from build123d import *

# Parameters (mm, degrees)
BOSS_EXTRUDE1_DEPTH = 15
DIAMETER_HOLE1_D    = 5.5
CHAMFER1_SIZE       = 5


with BuildPart() as part:
    # Sketch1 → Boss-Extrude1 (new body)
    with BuildSketch(Plane.XY):
        Polygon((-16, 36), (16, 36), (16, 10), (28, 10), (28, 0), (-28, 0), (-28, 10), (-16, 10), align=None)
    extrude(amount=-BOSS_EXTRUDE1_DEPTH)

    # Sketch2 → Cut-Revolve1 (revolve, cut)
    with BuildSketch(Plane(origin=(0, 0, 0), x_dir=(0, 0, -1), z_dir=(1, 0, 0)), mode=Mode.PRIVATE) as cut_revolve1_sk:
        Polygon((3.65, 32), (3.65, 32.6), (5, 32.6), (5, 32), (13, 32), (13, 30), (15, 30), (15, 20), (0, 20), (0, 32), align=None)
    revolve(cut_revolve1_sk.sketch.rotate(Axis((0, 20, -15), (0, 0, 1)), 90), axis=Axis((0, 20, -15), (0, 0, 1)), mode=Mode.SUBTRACT)

    # Diameter Hole1 (through all)
    with Locations(Plane(origin=(0, 10, 0), x_dir=(1, 0, 0), z_dir=(0, 1, 0))):
        with Locations((-22, 7.5), (22, 7.5)):
            Hole(DIAMETER_HOLE1_D / 2)

    # Chamfer1
    chamfer1_edges = [part.edges().sort_by_distance(p)[0] for p in [
        (-16, 36, -7.5),
        (16, 36, -7.5),
    ]]
    chamfer(chamfer1_edges, length=CHAMFER1_SIZE)


solid = part.part
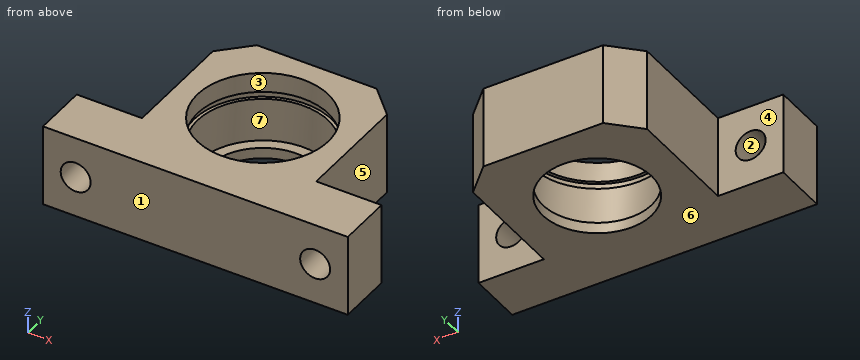
Can you work these out from the model? Positions are in its coordinate system, mm. Face numbers are marked on the shaded views. A direction names the side the tool comes from. Give positions to 0.01 mm unless a question says otherwise; leave off trailing zeros. Loops run counter-clockwise (first coordinate to the right, second up) from the corner with the lowest first, then second, coordinate; pieces in that order, holes last. Notation, with made-up numbers: (-14.75, 25.25) -> (-0.75, 25.25) arc R17 cw to (-0.75, 32.25) -> close; hole circle Ø3 at (28, 1). An arc over 180 degrees is marked (long way). Write item = value, one per line.
1) Suppose I cut it at D-D on y = 3.5. Write out the boundary of the cut face in (x, z).
Check result:
outline = (-28, -15) -> (28, -15) -> (28, 0) -> (-28, 0) -> close; hole circle Ø5.5 at (-22, -7.5); hole circle Ø5.5 at (22, -7.5)
2) Will these pins go through, and if not, where does the flat tip stop? pin 1 (6 mm diameter, centred on x = 24.5, z = -4.5, fed in from +Y); pin 2 (2 mm diameter, centred on y = 11.5, z = -5.5, fed in from -X); pin 3 (4 mm diameter, centred on y = 15.5, z = -5, fed in from +X).
Check result:
pin_1 = 10
pin_2 = -16
pin_3 = 16
3) Suppose I cut it at B-B on x = 22. Write out the boundary of the cut face in (y, z).
Check result:
outline = (0, -15) -> (10, -15) -> (10, -10.25) -> (0, -10.25) -> close; (0, -4.75) -> (10, -4.75) -> (10, 0) -> (0, 0) -> close
4) Suppose I cut it at A-A on z = -7.5. Write out the boundary of the cut face in (x, y).
Check result:
outline = (-28, 0) -> (-24.75, 0) -> (-24.75, 10) -> (-28, 10) -> close; (-19.25, 0) -> (19.25, 0) -> (19.25, 10) -> (16, 10) -> (16, 31) -> (11, 36) -> (-11, 36) -> (-16, 31) -> (-16, 10) -> (-19.25, 10) -> close; (24.75, 0) -> (28, 0) -> (28, 10) -> (24.75, 10) -> close; hole circle Ø24 at (0, 20)
5) For the marked faces 4, 5, 6 and 7, which set-ups out of +Z, -Z, +X, -X, +Y, -Y let a thin tool reach every point of the face, with its end or its side?
Check result:
face_4 = +Z, -Z, -X, +Y
face_5 = +Z, -Z, +X, +Y
face_6 = -Z, +X, -X, +Y, -Y
face_7 = +Z
6) Suppose I cut it at C-C on z = -2.25. Write out the boundary of the cut face in (x, y), then the cut area to 3 significant figures.
Check result:
outline = (-28, 0) -> (28, 0) -> (28, 10) -> (16, 10) -> (16, 31) -> (11, 36) -> (-11, 36) -> (-16, 31) -> (-16, 10) -> (-28, 10) -> close; hole circle Ø24 at (0, 20)
area = 915 mm2
7) I need wall thicknesses on L1, parallel to X at y = 20, z = -4.45; L2, parallel to Z at x = -22, y = 7; L3, parallel to X at y = 7.5, z = -6.25. Which ranges of each line are inside material? Lowest first, please. Write a range as from..to.
Check result:
L1 = -16..-12.6, 12.6..16
L2 = -15..-10.25, -4.75..0
L3 = -28..-24.45, -19.55..19.55, 24.45..28
8) Thinking about a two-plate mould opening in Y: for the marked faces 1, 2 and 3, which applies, released by +Y, released by -Y, zero draft, split by the parting line, or undercut?
Check result:
face_1 = released by -Y
face_2 = zero draft
face_3 = undercut
